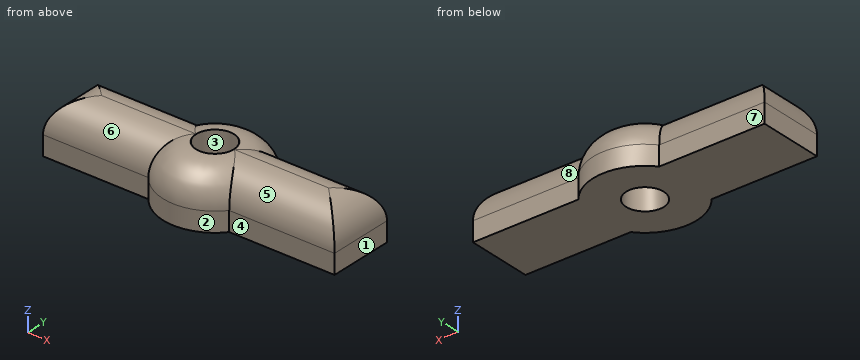
```python
from build123d import *

# Parameters (mm, degrees)
BOSS_EXTRU_2_DEPTH = 8
CONG_1_R           = 5
D_GAGEMENT_121_D   = 5.7912


with BuildPart() as part:
    # Esquisse1 → Boss.-Extru.2 (new body)
    with BuildSketch(Plane.XY):
        with BuildLine():
            Line((-22.5, 5), (-6.244997998, 5))
            ThreePointArc((-6.244997998, 5), (0, 8), (6.244997998, 5))
            Line((6.244997998, 5), (22.5, 5))
            Line((22.5, 5), (22.5, -5))
            Line((22.5, -5), (6.244997998, -5))
            ThreePointArc((6.244997998, -5), (0, -8), (-6.244997998, -5))
            Line((-6.244997998, -5), (-22.5, -5))
            Line((-22.5, -5), (-22.5, 5))
        make_face()
    extrude(amount=BOSS_EXTRU_2_DEPTH)

    # Congé1
    cong_1_edges = [part.edges().sort_by_distance(p)[0] for p in [
        (0, -8, 8),
        (14.372498999, -5, 8),
        (22.5, 0, 8),
        (14.372498999, 5, 8),
        (0, 8, 8),
        (-14.372498999, 5, 8),
        (-22.5, 0, 8),
        (-14.372498999, -5, 8),
    ]]
    fillet(cong_1_edges, radius=CONG_1_R - 0.0001)  # a hair under: the kernel refuses the full size

    # Dégagement #121 (through all)
    with Locations(Plane.XY.offset(8)):
        with Locations((0, 0)):
            Hole(D_GAGEMENT_121_D / 2)


solid = part.part
```
For this review, take the finished solid that the model builds, in its own axes (mm). Face numbers are marked on the shaded views. A direction names the side the tool comes from. Round coordinates to 2 decimals unless told otherwise and drop trailing zeros. Write each loop counter-clockwise with the first axis right and the second up, starting at its lowest first coordinate (ties: lowest second). Pieces come first, ordered by that corner, then holes. Notation, with made-up numbers: (-10.5, -36.5) - (15.5, -36.5) arc R34 ccw to (15.5, 1.5) - close; hole circle Ø5 at (-22.5, -5.5). An arc over 180 degrees is marked (long way). Answer as a JSON object with one key per item and string values.
1. We need section A-A on z = 1. Give the boundary of the cut face in (x, y) (3 decimals), then the cut area to 3 significant figures.
Response values:
{"outline": "(-22.5, -5) - (-6.245, -5) arc R8 ccw to (6.245, -5) - (22.5, -5) - (22.5, 5) - (6.245, 5) arc R8 ccw to (-6.245, 5) - (-22.5, 5) - close; hole circle Ø5.791 at (0, 0)", "area": "476 mm2"}
2. Tool access review of the marked faces 5, 6, 7 and 8: name each direction out of +Z, -Z, +X, -X, +Y, -Y from which nothing blocks a thin tool from reaching the whole face with its end or side.
Response values:
{"face 5": "+Z, +X, -Y", "face 6": "+Z, -X, -Y", "face 7": "+Z, -Z, -X, +Y", "face 8": "+Z, +X, +Y"}
3. We need section B-B on x = -18. Give the boundary of the cut face in (y, z), then the cut area to 3 significant figures.
Response values:
{"outline": "(-5, 0) - (5, 0) - (5, 3) arc R5 ccw to (0.5, 7.97) - (-0.5, 7.97) arc R5 ccw to (-5, 3) - close", "area": "69.3 mm2"}
4. For pin 1 Ø3.5 at (x, z) = (17, 1.5) entering from +Y; pin 2 Ø5 at (x, y) = (-12.5, 3) entering from +Z; pin 3 Ø1.5 at (x, z) = (-13, 1) entering from -Y, all flat-tipped, find the tip position at first contact; note any pin that passes through.
Response values:
{"pin 1": "stops at y = 5", "pin 2": "stops at z = 7.97", "pin 3": "stops at y = -5"}
5. Draft analysis for pull direction X (two halves, no side actions). For the marked faces 1, 2, 3 and 4, state which applies: +X half, -X half, draft (parallel to the pull), parting line (faces both ways), or undercut.
Response values:
{"face 1": "+X half", "face 2": "parting line", "face 3": "undercut", "face 4": "draft"}
6. To check wall thickness, follow line 1 along Y through (x, z) = (0, 1.5); line 2 along Y through (x, z) = (-13, 3.25); line 3 along Y through (x, z) = (0, 4.25). State the ranges of each line that lie inside material, in increasing order.
Response values:
{"line 1": "y = -8 to -2.9, 2.9 to 8", "line 2": "y = -4.99 to 4.99", "line 3": "y = -7.84 to -2.9, 2.9 to 7.84"}
